```python
from build123d import *

# Parameters (mm, degrees)
SKETCH1_W                 = 73.5
SKETCH1_H                 = 49.8
SLIDER_BODY_DEPTH         = 125
SKETCH2_R                 = 10.95
LEAD_NUT_INSET_DEPTH      = 15
SKETCH3_R                 = 6
LEADSCREW_CLEARANCE_DEPTH = 142.358728064
SKETCH9_W                 = 10
SKETCH9_H                 = 3
DECOUPLING_SLIT_DEPTH     = 154.320872682
BOLT_CLEARANCE_HOLES_D    = 6.6


with BuildPart() as part:
    # Sketch1 → slider body (new body)
    with BuildSketch(Plane.XY):
        with Locations((36.75, 24.9)):
            Rectangle(SKETCH1_W, SKETCH1_H)
    extrude(amount=SLIDER_BODY_DEPTH)

    # Sketch2 → lead nut inset (cut)
    with BuildSketch(Plane(origin=(0, 0, 0), x_dir=(-1, 0, 0), z_dir=(0, 0, -1))):
        with Locations((-36.75, 24.9)):
            Circle(SKETCH2_R)
    extrude(amount=-LEAD_NUT_INSET_DEPTH, mode=Mode.SUBTRACT)

    # Sketch3 → leadscrew clearance (cut, through all)
    with BuildSketch(Plane(origin=(0, 0, 15), x_dir=(-1, 0, 0), z_dir=(0, 0, -1))):
        with Locations((-36.75, 24.9)):
            Circle(SKETCH3_R)
    extrude(amount=-LEADSCREW_CLEARANCE_DEPTH, mode=Mode.SUBTRACT)

    # Sketch9 → decoupling slit (cut, through all)
    with BuildSketch(Plane.XZ):
        with Locations((68.5, 62.5)):
            Rectangle(SKETCH9_W, SKETCH9_H)
    decoupling_slit = extrude(amount=-DECOUPLING_SLIT_DEPTH, mode=Mode.SUBTRACT)

    # bolt clearance holes (through all)
    with Locations(Plane(origin=(0, 49.8, 0), x_dir=(1, 0, 0), z_dir=(0, 1, 0))):
        with Locations((51.75, -100), (21.75, -25), (51.75, -25), (21.75, -100), (21.75, -53), (51.75, -53)):
            Hole(BOLT_CLEARANCE_HOLES_D / 2)

    # mirror slit: decoupling slit across plane
    add(decoupling_slit.mirror(Plane.ZY.offset(-36.75)), mode=Mode.SUBTRACT)


solid = part.part
```
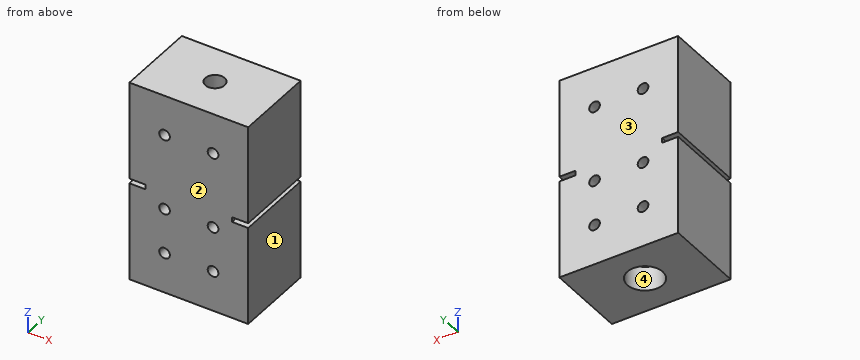
The model under review builds one solid part; all positions refer to its coordinate system, in mm. Face numbers are marked on the shaded views. Give positions to 0.01 mm unless a question says otherwise; leave off trailing zeros. Write each loop counter-clockwise with the first axis right and the second up, starting at its lowest first coordinate (ties: lowest second). Pieces come first, ordered by that corner, then holes.
(1) The part is to be moulded in two halves that separate along Y. For the marked faces 1, 2, 3 and 4, say which applies: released by +Y, released by -Y, zero draft, split by the parting line, or undercut.
(2) Consider section C-C, the plane x = 36.75. Give the boundary of the cut face in (y, z).
(3) To check wall thickness, follow L1, parallel to Z at x = 51.75, y = 32; L2, parallel to X at y = 37, z = 25; L3, parallel to Z at x = 49, y = 35.5. State the ranges of each line that lie inside material, in increasing order.
(4) Consider section A-A, the plane y = 24.9. Give the boundary of the cut face in (x, z).
(5) Consider section D-D, the plane x = 21.75. Give the boundary of the cut face in (y, z), and give its area (3 significant figures).
(6) Consider section B-B, the plane z = 100. Give the boundary of the cut face in (x, y), and give its area (3 significant figures).
(7) For P1, Ø6, axis at x = 21.75, z = 100, coming from the -Y side; P2, Ø6.5, axis at x = 38, y = 21, coming from the -Z side; P3, Ø1.5, axis at y = 15, z = 62.5, coming from the -X side; P4, Ø0.9, axis at y = 36.5, z = 62, coming from the +X side, all flat-tipped, find the tip position at first contact; note any pin that passes through.
Returned:
1. face 1: zero draft
1. face 2: released by -Y
1. face 3: released by +Y
1. face 4: undercut
2. outline: (0, 0) - (13.95, 0) - (13.95, 15) - (18.9, 15) - (18.9, 125) - (0, 125) - close; (30.9, 15) - (35.85, 15) - (35.85, 0) - (49.8, 0) - (49.8, 125) - (30.9, 125) - close
3. L1: z = 0 to 21.7, 28.3 to 49.7, 56.3 to 96.7, 103.3 to 125
3. L2: x = 0 to 18.45, 25.05 to 48.45, 55.05 to 73.5
3. L3: z = 0 to 23.18, 26.82 to 51.18, 54.82 to 98.18, 101.82 to 125
4. outline: (0, 0) - (25.8, 0) - (25.8, 15) - (30.75, 15) - (30.75, 125) - (0, 125) - (0, 64) - (10, 64) - (10, 61) - (0, 61) - close; (42.75, 15) - (47.7, 15) - (47.7, 0) - (73.5, 0) - (73.5, 61) - (63.5, 61) - (63.5, 64) - (73.5, 64) - (73.5, 125) - (42.75, 125) - close; hole circle Ø6.6 at (21.75, 25); hole circle Ø6.6 at (21.75, 53); hole circle Ø6.6 at (21.75, 100); hole circle Ø6.6 at (51.75, 25); hole circle Ø6.6 at (51.75, 53); hole circle Ø6.6 at (51.75, 100)
5. outline: (0, 0) - (49.8, 0) - (49.8, 21.7) - (0, 21.7) - close; (0, 28.3) - (49.8, 28.3) - (49.8, 49.7) - (0, 49.7) - close; (0, 56.3) - (49.8, 56.3) - (49.8, 96.7) - (0, 96.7) - close; (0, 103.3) - (49.8, 103.3) - (49.8, 125) - (0, 125) - close
5. area: 5,240 mm2
6. outline: (0, 0) - (18.45, 0) - (18.45, 49.8) - (0, 49.8) - close; (25.05, 0) - (48.45, 0) - (48.45, 49.8) - (25.05, 49.8) - close; (55.05, 0) - (73.5, 0) - (73.5, 49.8) - (55.05, 49.8) - close; hole circle Ø12 at (36.75, 24.9)
6. area: 2,890 mm2
7. P1: passes through
7. P2: stops at z = 15
7. P3: stops at x = 10
7. P4: stops at x = 63.5
